Part print with two shaded views. Sizes in mm from the minimum x, y, z corner. A direction names the side the tool comes from. Round coordinates to 2 decimals unless told otherwise and drop trailing zeros. Write each loop counter-clockwise with the first axis right and the second up, starting at its lowest first coordinate (ties: lowest second). Pieces come first, ordered by that corner, then holes. Notation, with made-up numbers: (-37, -3.75) -> (-28, -3.75) arc R9 ccw to (-28, 13.25) -> close; hole circle Ø4 at (-22.75, 70). An arc over 180 degrees is marked (long way). Return JSON: item names as keys, results as strings.
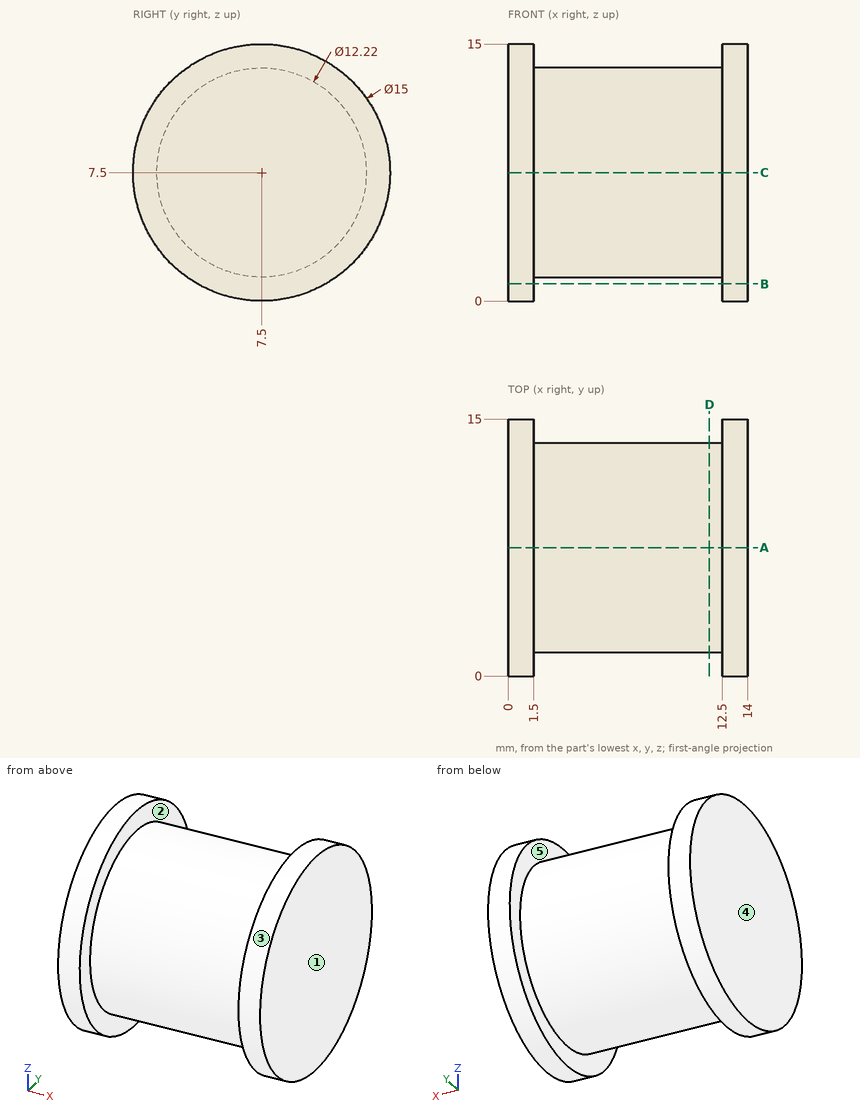
Q1. 3-axis set-ups, long thin cutter, end or side, ignore diameter. For the marked faces 1 and 2: which of +Z, -Z, +X, -X, +Y, -Y reach the whole face in a straight line?
Verdict:
{"face 1": "+Z, -Z, +X, +Y, -Y", "face 2": "none"}
Q2. Pin check, flat tips, straight feed: pin 1 Ø3 at (x, z) = (12.5, 4) entering from -Y; pin 2 Ø5 at (x, y) = (6.5, 7) entering from +Z. Stop position of each tip, or through.
Verdict:
{"pin 1": "stops at y = 0.27", "pin 2": "stops at z = 13.61"}
Q3. Saw through at D-D on x = 11.75. List the corners of the cut face in (y, z), then the cut area to 3 significant figures.
Verdict:
{"outline": "circle Ø12.22 at (7.5, 7.5)", "area": "117 mm²"}
Q4. Saw through at A-A on y = 7.5. List the corners of the cut face in (x, z).
Verdict:
{"outline": "(0, 0) -> (1.5, 0) -> (1.5, 1.39) -> (12.5, 1.39) -> (12.5, 0) -> (14, 0) -> (14, 15) -> (12.5, 15) -> (12.5, 13.61) -> (1.5, 13.61) -> (1.5, 15) -> (0, 15) -> close"}
Q5. Saw through at B-B on z = 1. List the corners of the cut face in (x, y), then the cut area to 4 significant figures.
Verdict:
{"outline": "(0, 3.76) -> (1.5, 3.76) -> (1.5, 11.24) -> (0, 11.24) -> close; (12.5, 3.76) -> (14, 3.76) -> (14, 11.24) -> (12.5, 11.24) -> close", "area": "22.45 mm²"}
Q6. Two-plate mould, pull along X, no slides. Class the marked faces 3, 4 and 5: +X half, -X half, draft (parallel to the pull), parting line (faces both ways), or undercut.
Verdict:
{"face 3": "draft", "face 4": "-X half", "face 5": "undercut"}
Q7. Wall check: L1, parallel to X at y = 14.25, z = 9.5; L2, parallel to Y at x = 2.75, z = 7.75; L3, parallel to Z at x = 12.75, y = 7.75. Give the ranges that are in metal, low to high.
Verdict:
{"L1": "x = 0 to 1.5, 12.5 to 14", "L2": "y = 1.4 to 13.6", "L3": "z = 0 to 15"}
